Verification items for this drawing (mm, ordinates from the low corner). A direction names the side the tool comes from. Round coordinates to 2 decimals unless told otherwise and drop trailing zeros. Loops run counter-clockwise (first coordinate to the right, second up) from the corner with the lowest first, then second, coordinate; pieces in that order, holes last. Notation, with made-up numbers: M 13.25,69.5 L 25.25,69.5 A11 ccw 25.25,89.5 Z; hole C -16.5,-37.5 d8. An arc over 180 degrees is marked long. Write item = value, one per line.
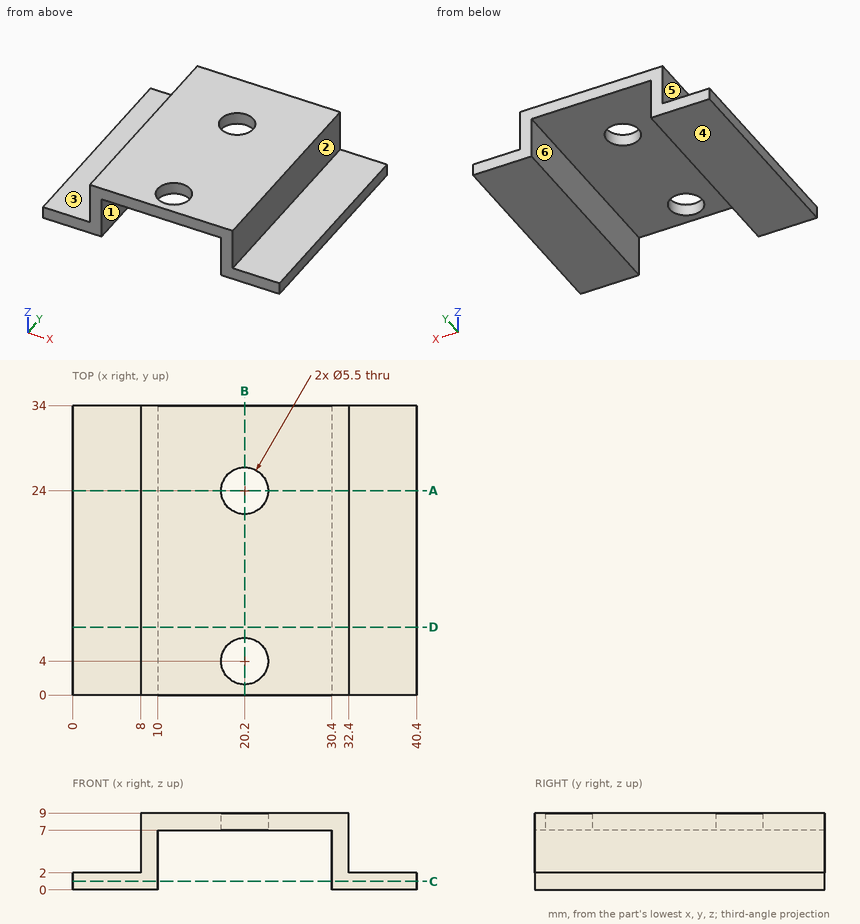
(1) Material ranges on line 1 along Y through (x, z) = (20.2, 8.6); line 2 along X through (y, z) = (18.5, 2.25); line 3 along X through (y, z) = (12, 1.5), recorded low to high. Write a range as from..to.
Result set:
line_1 = 0..1.25, 6.75..21.25, 26.75..34
line_2 = 8..10, 30.4..32.4
line_3 = 0..10, 30.4..40.4
(2) Sectioned sample at B-B on x = 20.2. Record the cut outline in (y, z), then the cut area to 3 significant figures.
Result set:
outline = M 0,7 L 1.25,7 L 1.25,9 L 0,9 Z; M 6.75,7 L 21.25,7 L 21.25,9 L 6.75,9 Z; M 26.75,7 L 34,7 L 34,9 L 26.75,9 Z
area = 46.0 mm2
(3) Sectioned sample at C-C on z = 1. Record the cut outline in (x, y), then the cut area to 3 significant figures.
Result set:
outline = M 0,0 L 10,0 L 10,34 L 0,34 Z; M 30.4,0 L 40.4,0 L 40.4,34 L 30.4,34 Z
area = 680 mm2
(4) Sectioned sample at D-D on y = 8. Record the cut outline in (x, z).
Result set:
outline = M 0,0 L 10,0 L 10,7 L 30.4,7 L 30.4,0 L 40.4,0 L 40.4,2 L 32.4,2 L 32.4,9 L 8,9 L 8,2 L 0,2 Z
(5) Depth check by flat-ended pin: pin 1 Ø3 at (x, y) = (15.5, 10.5) entering from -Z; pin 2 Ø9 at (x, y) = (38, 14) entering from +Z; pin 3 Ø3 at (y, z) = (7.5, 5.5) entering from +X; pin 4 Ø4 at (x, z) = (4.5, 1) entering from -Y. Enter the tip coordinate at first touch or a pass-through.
Result set:
pin_1 = 7
pin_2 = 2
pin_3 = 32.4
pin_4 = 0
(6) Tool access check on the marked faces 1, 2 and 3. Record the directions out of +Z, -Z, +X, -X, +Y, -Y that give a thin tool (end or side, any length) a straight path to the whole face; none if there is none.
Result set:
face_1 = -Z, +Y, -Y
face_2 = +Z, +X, +Y, -Y
face_3 = +Z, -X, +Y, -Y
(7) Release check for a two-part mould opening along X. For the marked faces 4, 5 and 6 record: released by +X, released by -X, zero draft, split by the parting line, or undercut.
Result set:
face_4 = zero draft
face_5 = released by -X
face_6 = undercut
(8) Sectioned sample at A-A on y = 24. Record the cut outline in (x, z), then the cut area to 3 significant figures.
Result set:
outline = M 0,0 L 10,0 L 10,7 L 17.45,7 L 17.45,9 L 8,9 L 8,2 L 0,2 Z; M 22.95,7 L 30.4,7 L 30.4,0 L 40.4,0 L 40.4,2 L 32.4,2 L 32.4,9 L 22.95,9 Z
area = 97.8 mm2
